from build123d import *
from OCP.BRepFilletAPI import BRepFilletAPI_MakeChamfer

# Parameters (mm, degrees)
SKETCH_1_W              = 67
SKETCH_1_H              = 48
EXTRUDE_1_DEPTH         = 1.6
FILLET_1_R              = 4
HOLE_WIZARD_3_2_3_2_1_D = 3.2
SKETCH_4_W              = 6.8
SKETCH_4_H              = 6.8
SKETCH_4_W_2            = 3.2
SKETCH_4_H_2            = 5
SKETCH_4_W_3            = 6.5
SKETCH_4_H_3            = 3.5
EXTRUDE_2_DEPTH         = 1.6
SKETCH_5_W              = 52
SKETCH_5_H              = 8
EXTRUDE_4_DEPTH         = 10
CHAMFER_1_SIZE          = 3
CHAMFER_1_SIZE2         = 1.732050808
SKETCH_7_W              = 6
SKETCH_7_H              = 4
EXTRUDE_5_DEPTH         = 3


with BuildPart() as part:
    # 草图1 → 凸台-拉伸1 (new body)
    with BuildSketch(Plane(origin=(0, 0, 0), x_dir=(1, 0, 0), z_dir=(0, 1, 0))):
        with Locations((33.5, 24)):
            Rectangle(SKETCH_1_W, SKETCH_1_H)
    extrude(amount=EXTRUDE_1_DEPTH)

    # 圆角1
    fillet_1_edges = [part.edges().sort_by_distance(p)[0] for p in [
        (0, 0.8, -48),
        (67, 0.8, -48),
        (67, 0.8, 0),
        (0, 0.8, 0),
    ]]
    fillet(fillet_1_edges, radius=FILLET_1_R)

    # Ø3.2 (3.2) 直径孔1 (through all)
    with Locations(Plane(origin=(0, 1.6, 0), x_dir=(1, 0, 0), z_dir=(0, 1, 0))):
        with Locations((4, 9), (4, 42), (63, 42), (63, 9)):
            Hole(HOLE_WIZARD_3_2_3_2_1_D / 2)

    # 草图4 → 凸台-拉伸2 (add)
    with BuildSketch(Plane(origin=(0, 1.6, 0), x_dir=(1, 0, 0), z_dir=(0, 1, 0))):
        with Locations((39.4, 22.4)):
            Rectangle(SKETCH_4_W, SKETCH_4_H)
        with Locations((26.8, 25)):
            Rectangle(SKETCH_4_W_2, SKETCH_4_H_2)
        with Locations((12.75, 19.25)):
            Rectangle(SKETCH_4_W_3, SKETCH_4_H_3)
    extrude(amount=EXTRUDE_2_DEPTH)

    # 草图5 → 凸台-拉伸4 (add)
    with BuildSketch(Plane(origin=(0, 1.6, 0), x_dir=(1, 0, 0), z_dir=(0, 1, 0))):
        with Locations((33.5, 4.2)):
            Rectangle(SKETCH_5_W, SKETCH_5_H)
    extrude(amount=EXTRUDE_4_DEPTH)

    # 倒角1: one chamfer whose edges measure the first distance from different faces: ONE call of the kernel's chamfer builder (chamfer() names one face for all edges)
    chamfer_1_edges_1 = [part.edges().sort_by_distance(p)[0] for p in [
        (33.5, 11.6, -0.2),
    ]]
    chamfer_1_side_1 = [part.faces().sort_by_distance(p)[0] for p in [
        (33.5, 6.6, -0.2),
    ]]
    chamfer_1_edges_2 = [part.edges().sort_by_distance(p)[0] for p in [
        (33.5, 11.6, -8.2),
    ]]
    chamfer_1_side_2 = [part.faces().sort_by_distance(p)[0] for p in [
        (33.5, 6.6, -8.2),
    ]]
    chamfer_1 = BRepFilletAPI_MakeChamfer(part.part.solid().wrapped)
    for e in chamfer_1_edges_1:
        chamfer_1.Add(CHAMFER_1_SIZE, CHAMFER_1_SIZE2, e.wrapped, chamfer_1_side_1[0].wrapped)  # the first distance lies on this face
    for e in chamfer_1_edges_2:
        chamfer_1.Add(CHAMFER_1_SIZE, CHAMFER_1_SIZE2, e.wrapped, chamfer_1_side_2[0].wrapped)  # the first distance lies on this face
    add(Compound.cast(chamfer_1.Shape()), mode=Mode.REPLACE)

    # 草图7 → 凸台-拉伸5 (add)
    with BuildSketch(Plane(origin=(0, 1.6, 0), x_dir=(1, 0, 0), z_dir=(0, 1, 0))):
        with Locations((16.5, 35.5)):
            Rectangle(SKETCH_7_W, SKETCH_7_H)
        with Locations((36.5, 35.5)):
            Rectangle(SKETCH_7_W, SKETCH_7_H)
    extrude(amount=EXTRUDE_5_DEPTH)


solid = part.part
The listing builds one solid part. Answer for the finished solid, in the listing's coordinates (mm). A direction names the side the tool comes from. Give positions to 0.01 mm unless a question says otherwise; leave off trailing zeros. Loops run counter-clockwise (first coordinate to the right, second up) from the corner with the lowest first, then second, coordinate; pieces in that order, holes last. Notation, with made-up numbers: (-19.5, 30.5) - (9.5, 30.5) arc R21 cw to (9.5, 54.5) - close; hole circle Ø1 at (-25.5, -5). An arc over 180 degrees is marked (long way). Answer as a JSON object with one key per item and string values.
1. For faces 4 (the flat face through (42.8, 2, -22)), 5 (the flat face through (25.2, 2, -25)), 6 (the flat face through (33, 5, -8.2)), 7 (the flat face through (27, 2, -22.5)), determine the directions among +Z, -Z, +X, -X, +Y, -Y from which every point of the face is accessible in a straight line to the end or side of a thin tool.
Determined:
{"face 4": "-Z, +X, +Y", "face 5": "-Z, -X, +Y", "face 6": "+X, -X, +Y", "face 7": "-X, +Y"}
2. A cutting plane is placed at C-C (x = 11.5). Write down the section's boundary in (y, z).
Determined:
{"outline": "(0, -48) - (1.6, -48) - (1.6, -21) - (3.2, -21) - (3.2, -17.5) - (1.6, -17.5) - (1.6, -8.2) - (8.6, -8.2) - (11.6, -6.47) - (11.6, -1.93) - (8.6, -0.2) - (1.6, -0.2) - (1.6, 0) - (0, 0) - close"}
3. Flat-ended cylindrical pins translate along their axes: pin 1 Ø1.5 at (x, y) = (13.5, 5) entering from +Z; pin 2 Ø5.5 at (x, y) = (42.5, 6.5) entering from -Z; pin 3 Ø4 at (y, z) = (8, -4.5) entering from -X; pin 4 Ø1.9 at (x, z) = (63, -9) entering from -Y. Find the tip coordinate at first contact, or state that the pin passes through.
Determined:
{"pin 1": "z = -0.2", "pin 2": "z = -8.2", "pin 3": "x = 7.5", "pin 4": "through"}
4. A cutting plane is placed at A-A (y = 2.5). Write down the section's boundary in (x, z), then the cut area to 3 significant figures.
Determined:
{"outline": "(7.5, -8.2) - (59.5, -8.2) - (59.5, -0.2) - (7.5, -0.2) - close; (9.5, -21) - (16, -21) - (16, -17.5) - (9.5, -17.5) - close; (13.5, -37.5) - (19.5, -37.5) - (19.5, -33.5) - (13.5, -33.5) - close; (25.2, -27.5) - (28.4, -27.5) - (28.4, -22.5) - (25.2, -22.5) - close; (33.5, -37.5) - (39.5, -37.5) - (39.5, -33.5) - (33.5, -33.5) - close; (36, -25.8) - (42.8, -25.8) - (42.8, -19) - (36, -19) - close", "area": "549 mm²"}
5. For a pull along Z with two mould halves and no side action, classify faces 1 (the flat face through (36, 4.6, -36)), 2 (the flat face through (13, 2, -17.5)), 3 (the flat face through (33.136, 10.121, -7.322)) as pulls with the +Z half, pulls with the -Z half, needs draft (parallel to the pull), parting line crosses it, or undercut.
Determined:
{"face 1": "needs draft", "face 2": "undercut", "face 3": "pulls with the -Z half"}
6. A cutting plane is placed at D-D (z = -14). Write down the section's boundary in (x, y).
Determined:
{"outline": "(0, 0) - (67, 0) - (67, 1.6) - (0, 1.6) - close"}
7. Find the intervals of material crossed by L1, parallel to Z at x = 4, y = 1.05; L2, parallel to X at y = 0.75, z = -42; L3, parallel to Y at x = 28, z = -41.5, in increasing order. Write a range as [from, to].
Determined:
{"L1": "[-48, -43.6], [-40.4, -10.6], [-7.4, 0]", "L2": "[0, 2.4], [5.6, 61.4], [64.6, 67]", "L3": "[0, 1.6]"}
8. A cutting plane is placed at B-B (z = -42). Write down the section's boundary in (x, y), then the cut area to 3 significant figures.
Determined:
{"outline": "(0, 0) - (2.4, 0) - (2.4, 1.6) - (0, 1.6) - close; (5.6, 0) - (61.4, 0) - (61.4, 1.6) - (5.6, 1.6) - close; (64.6, 0) - (67, 0) - (67, 1.6) - (64.6, 1.6) - close", "area": "97.0 mm²"}
